Work out the finished part from the listing and answer in its coordinate system (mm). Face numbers are marked on the shaded views. A direction names the side the tool comes from. Coordinates: 2 decimals unless noted, no trailing zeros. Write each loop counter-clockwise with the first axis right and the second up, starting at its lowest first coordinate (ties: lowest second). Pieces come first, ordered by that corner, then holes. Notation, with made-up numbers: (48, 86.25) - (81, 86.25) arc R28 cw to (81, 113.25) - close; hole circle Ø9 at (13.25, -7.75). An arc over 180 degrees is marked (long way). Use a Markdown table: item, result. Add a question column.
(1) The part is cut by section A-A, the plane y = -21. Give the vertices of the cut face in (x, z) (1 decimal).
(2) Given pin 1 Ø3 at (y, z) = (-6, 25.5) entering from +X; pin 2 Ø10 at (y, z) = (-16, 13.5) entering from +X; pin 3 Ø12 at (y, z) = (-15, 21) entering from -X; pin 4 Ø8 at (x, z) = (19.5, 11) entering from +Y, each flat-ended and moving along its own axis, determine where each tip first touches the part or whether it passes through.
(3) The part is cut by section D-D, the plane z = 11. Give the vertices of the cut face in (x, y), then the cut area to 3 significant figures.
(4) The part is cut by section C-C, the plane x = 39.5. Give the vertices of the cut face in (y, z), then the cut area to 3 significant figures.
(5) For a pull along X with two mould halves and no side action, classify the marked faces 1, 2 and 3 as released by +X, released by -X, zero draft, split by the parting line, or undercut.
(6) The part is cut by section B-B, the plane z = 14. Give the vertices of the cut face in (x, y), then the cut area to 3 significant figures.
(7) Find the intervals of material crossed by line 1 (Z direction, x = 36, y = -9.75); line 2 (X direction, y = -9.25, z = 11.25) (3 decimals); line 3 (X direction, y = -23.5, z = 17), in increasing order. Write a range as from..to.
(8) A tool of negligible diameter and unlimited length cuts with its end or side. For the marked faces 4 and 5, from which of +Z, -Z, +X, -X, +Y, -Y can it reach the whole face along a straight path? Write none if from no direction.
from build123d import *

# Parameters (mm, degrees)
F1_DEPTH = 25
F2_SIZE  = 2
F3_R     = 3


with BuildPart() as f1:
    # F0 (on Front) → F1 (new body)
    with BuildSketch(Plane.XZ):
        Polygon((-5, 30), (-10, 0), (56, 0), (51, 30), (46, 30), (46, 25), (46, 6), (0, 6), (0, 25), (0, 30), align=None)
        with BuildLine():
            ThreePointArc((0, 25), (2, 27.5), (0, 30))
            Line((0, 30), (0, 25))
        make_face()
        with BuildLine():
            Line((46, 25), (46, 30))
            ThreePointArc((46, 30), (44, 27.5), (46, 25))
        make_face()
    extrude(amount=F1_DEPTH)

    # F2
    f2_edges = [f1.edges().sort_by_distance(p)[0] for p in [
        (46, -12.5, 6),
        (0, -12.5, 6),
    ]]
    chamfer(f2_edges, length=F2_SIZE)

    # F3
    f3_edges = [f1.edges().sort_by_distance(p)[0] for p in [
        (51, -12.5, 30),
        (-5, -12.5, 30),
    ]]
    fillet(f3_edges, radius=F3_R)


solid = f1.part
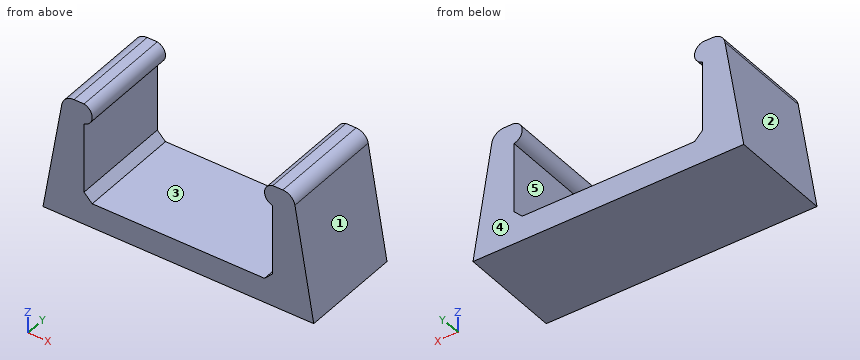
Model answer:
| question | item | result |
|---|---|---|
| 1 | outline | (-10, 0) - (56, 0) - (51.4, 27.5) arc R3 ccw to (48.5, 30) - (46, 30) arc R2.6 ccw to (46, 25) - (46, 8) - (44, 6) - (2, 6) - (0, 8) - (0, 25) arc R2.6 ccw to (0, 30) - (-2.5, 30) arc R3 ccw to (-5.4, 27.5) - close |
| 2 | pin 1 | x = 52 |
| 2 | pin 2 | x = 54.58 |
| 2 | pin 3 | x = -7.5 |
| 2 | pin 4 | through |
| 3 | outline | (-8.17, -25) - (0, -25) - (0, 0) - (-8.17, 0) - close; (46, -25) - (54.17, -25) - (54.17, 0) - (46, 0) - close |
| 3 | area | 408 mm^2 |
| 4 | outline | (-25, 0) - (0, 0) - (0, 6) - (-25, 6) - close |
| 4 | area | 150 mm^2 |
| 5 | face 1 | released by +X |
| 5 | face 2 | released by -X |
| 5 | face 3 | undercut |
| 6 | outline | (-7.67, -25) - (0, -25) - (0, 0) - (-7.67, 0) - close; (46, -25) - (53.67, -25) - (53.67, 0) - (46, 0) - close |
| 6 | area | 383 mm^2 |
| 7 | line 1 | 0..6 |
| 7 | line 2 | -8.125..0, 46..54.125 |
| 7 | line 3 | -7.17..0, 46..53.17 |
| 8 | face 4 | +Z, -Z, +X, -X, +Y |
| 8 | face 5 | +Y, -Y |
